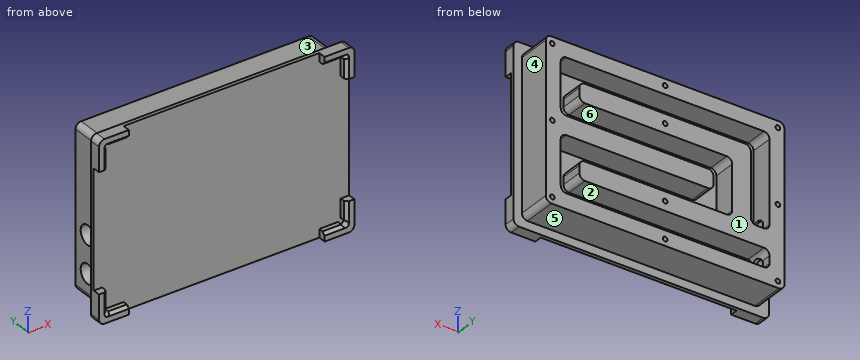
```python
from build123d import *

# Parameters (mm, degrees)
SKETCH1_W                         = 128
SKETCH1_H                         = 85.7
BOSS_EXTRUDE1_DEPTH               = 18
CUT_EXTRUDE1_DEPTH                = 12
M3X0_5_TAPPED_HOLE1_D             = 2.5
M3X0_5_TAPPED_HOLE1_DEPTH         = 10
M3X0_5_TAPPED_HOLE1_TIP           = 0.751075774
SKETCH10_W                        = 137
SKETCH10_H                        = 94.7
BOSS_EXTRUDE2_DEPTH               = 6
CUT_EXTRUDE2_DEPTH                = 4
SKETCH12_W                        = 4.5
SKETCH12_H                        = 62.7
SKETCH12_W_2                      = 105
SKETCH12_H_2                      = 4.475
CUT_EXTRUDE3_DEPTH                = 4
CHAMFER1_SIZE                     = 1.5
FILLET1_R                         = 3
F_1_8_NPT_TAPPED_HOLE1_AT_2_COUNT = 2
F_1_8_NPT_TAPPED_HOLE1_AT_2_PITCH = 19.935714286


with BuildPart() as part:
    # Sketch1 → Boss-Extrude1 (new body)
    with BuildSketch(Plane(origin=(0, 0, 0), x_dir=(1, 0, 0), z_dir=(0, 1, 0))):
        Rectangle(SKETCH1_W, SKETCH1_H)
    extrude(amount=BOSS_EXTRUDE1_DEPTH)

    # Sketch2 → Cut-Extrude1 (cut)
    with BuildSketch(Plane(origin=(0, 18, 0), x_dir=(1, 0, 0), z_dir=(0, 1, 0))):
        with BuildLine():
            Line((-46, 11.935714286), (-46, -21.892857143))
            ThreePointArc((-46, -21.892857143), (-45.121320344, -24.014177486), (-43, -24.892857143))
            Line((-43, -24.892857143), (43, -24.892857143))
            ThreePointArc((43, -24.892857143), (45.121320344, -24.014177486), (46, -21.892857143))
            Line((46, -21.892857143), (46, -17.935714286))
            ThreePointArc((46, -17.935714286), (45.121320344, -15.814393942), (43, -14.935714286))
            Line((43, -14.935714286), (-33, -14.935714286))
            ThreePointArc((-33, -14.935714286), (-35.121320344, -14.057034629), (-36, -11.935714286))
            Line((-36, -11.935714286), (-36, 11.935714286))
            ThreePointArc((-36, 11.935714286), (-35.121320344, 14.057034629), (-33, 14.935714286))
            Line((-33, 14.935714286), (43, 14.935714286))
            ThreePointArc((43, 14.935714286), (45.121320344, 15.814393942), (46, 17.935714286))
            Line((46, 17.935714286), (46, 21.892857143))
            ThreePointArc((46, 21.892857143), (45.121320344, 24.014177486), (43, 24.892857143))
            Line((43, 24.892857143), (-53, 24.892857143))
            ThreePointArc((-53, 24.892857143), (-55.121320344, 25.771536799), (-56, 27.892857143))
            Line((-56, 27.892857143), (-56, 31.85))
            ThreePointArc((-56, 31.85), (-55.121320344, 33.971320344), (-53, 34.85))
            Line((-53, 34.85), (53, 34.85))
            ThreePointArc((53, 34.85), (55.121320344, 33.971320344), (56, 31.85))
            Line((56, 31.85), (56, 7.978571429))
            ThreePointArc((56, 7.978571429), (55.121320344, 5.857251085), (53, 4.978571429))
            Line((53, 4.978571429), (-23, 4.978571429))
            ThreePointArc((-23, 4.978571429), (-25.121320344, 4.099891772), (-26, 1.978571429))
            Line((-26, 1.978571429), (-26, -1.978571429))
            ThreePointArc((-26, -1.978571429), (-25.121320344, -4.099891772), (-23, -4.978571429))
            Line((-23, -4.978571429), (53, -4.978571429))
            ThreePointArc((53, -4.978571429), (55.121320344, -5.857251085), (56, -7.978571429))
            Line((56, -7.978571429), (56, -31.85))
            ThreePointArc((56, -31.85), (55.121320344, -33.971320344), (53, -34.85))
            Line((53, -34.85), (-53, -34.85))
            ThreePointArc((-53, -34.85), (-55.121320344, -33.971320344), (-56, -31.85))
            Line((-56, -31.85), (-56, 11.935714286))
            ThreePointArc((-56, 11.935714286), (-55.121320344, 14.057034629), (-53, 14.935714286))
            Line((-53, 14.935714286), (-49, 14.935714286))
            ThreePointArc((-49, 14.935714286), (-46.878679656, 14.057034629), (-46, 11.935714286))
        make_face()
    extrude(amount=-CUT_EXTRUDE1_DEPTH, mode=Mode.SUBTRACT)

    # M3x0.5 Tapped Hole1
    with Locations(Plane(origin=(0, 18, 0), x_dir=(1, 0, 0), z_dir=(0, 1, 0))):
        with Locations((-60.5, 39.35), (0, 39.35), (60.5, 39.35), (60.5, 0), (60.5, -39.35), (0, -39.35), (-60.5, -39.35), (-60.5, 0), (0, 19.914285714), (0, -19.914285714)):
            Hole(M3X0_5_TAPPED_HOLE1_D / 2, depth=M3X0_5_TAPPED_HOLE1_DEPTH)
            with Locations((0, 0, -(M3X0_5_TAPPED_HOLE1_DEPTH + M3X0_5_TAPPED_HOLE1_TIP / 2))):  # 118° drill point
                Cone(0, M3X0_5_TAPPED_HOLE1_D / 2, M3X0_5_TAPPED_HOLE1_TIP, mode=Mode.SUBTRACT)

    # Sketch10 → Boss-Extrude2 (add)
    with BuildSketch(Plane.XZ):
        Rectangle(SKETCH10_W, SKETCH10_H)
    extrude(amount=BOSS_EXTRUDE2_DEPTH)

    # Sketch11 → Cut-Extrude2 (cut)
    with BuildSketch(Plane.XZ.offset(6)):
        with BuildLine():
            Line((-62.5, -42.875), (62.5, -42.875))
            ThreePointArc((62.5, -42.875), (65.060660172, -43.935660172), (64, -41.375))
            Line((64, -41.375), (64, 41.375))
            ThreePointArc((64, 41.375), (65.060660172, 43.935660172), (62.5, 42.875))
            Line((62.5, 42.875), (-62.5, 42.875))
            ThreePointArc((-62.5, 42.875), (-65.060660172, 43.935660172), (-64, 41.375))
            Line((-64, 41.375), (-64, -41.375))
            ThreePointArc((-64, -41.375), (-65.060660172, -43.935660172), (-62.5, -42.875))
        make_face()
    extrude(amount=-CUT_EXTRUDE2_DEPTH, mode=Mode.SUBTRACT)

    # Sketch12 → Cut-Extrude3 (cut)
    with BuildSketch(Plane.XZ.offset(6)):
        with Locations((-66.25, 0)):
            Rectangle(SKETCH12_W, SKETCH12_H)
        with Locations((66.25, 0)):
            Rectangle(SKETCH12_W, SKETCH12_H)
        with Locations((0, 45.1125)):
            Rectangle(SKETCH12_W_2, SKETCH12_H_2)
        with Locations((0, -45.1125)):
            Rectangle(SKETCH12_W_2, SKETCH12_H_2)
    extrude(amount=-CUT_EXTRUDE3_DEPTH, mode=Mode.SUBTRACT)

    # Chamfer1
    chamfer1_edges = [part.edges().sort_by_distance(p)[0] for p in [
        (-64, -6, 36.3625),
        (-57.5, -6, -42.875),
        (64, -6, -36.3625),
        (57.5, -6, 42.875),
        (-64, -6, -36.3625),
        (57.5, -6, -42.875),
        (64, -6, 36.3625),
        (-57.5, -6, 42.875),
    ]]
    chamfer(chamfer1_edges, length=CHAMFER1_SIZE - 0.0001)  # a hair under: the kernel refuses the full size

    # Fillet1
    fillet1_edges = [part.edges().sort_by_distance(p)[0] for p in [
        (-68.5, -3, -47.35),
        (68.5, -3, -47.35),
        (68.5, -3, 47.35),
        (-68.5, -3, 47.35),
        (64, 9, 42.85),
        (-64, 9, 42.85),
        (-64, 9, -42.85),
        (64, 9, -42.85),
    ]]
    fillet(fillet1_edges, radius=FILLET1_R)

    # Sketch14 → 1/8 NPT Tapped Hole1 (revolve, cut)
    with BuildSketch(Plane(origin=(-64, 9, -29.871428571), x_dir=(0, 0, 1), z_dir=(0, 1, 0))):
        Polygon((0, 0), (0, 14.153468714), (4.2164, 11.62), (4.2164, 6.92), (4.936178933, 6.92), (5.143373, 0), align=None)
    f_1_8_npt_tapped_hole1 = revolve(axis=Axis((-70.35, 9, -29.871428571), (1, 0, 0)), mode=Mode.SUBTRACT)

    # 1/8 NPT Tapped Hole1 at 2: 1/8 NPT Tapped Hole1 ×2
    with Locations(*[(0, 0, i * F_1_8_NPT_TAPPED_HOLE1_AT_2_PITCH) for i in range(1, F_1_8_NPT_TAPPED_HOLE1_AT_2_COUNT)]):
        add(f_1_8_npt_tapped_hole1, mode=Mode.SUBTRACT)


solid = part.part
```
Input: part model. Units: mm. Frame: model coordinates. Face numbers are marked on the shaded views. A direction names the side the tool comes from. Coordinates: 2 decimals unless noted, no trailing zeros. Write each loop counter-clockwise with the first axis right and the second up, starting at its lowest first coordinate (ties: lowest second). Pieces come first, ordered by that corner, then holes.
1) Section A-A on x = 22.5. Output: boundary loops of the cut face in (y, z).
2) Section C-C on x = -29. Output: boundary loops of the cut face in (y, z), and give its area (3 significant figures).
3) Section B-B on y = 15.5. State how many separate pieces and enclosed holes the cut face has, and give its area (3 significant figures).
4) Set-up query: the marked faces 1 and 2. Return all of +Z, -Z, +X, -X, +Y, -Y with unobstructed straight access to the full face (end or side cutting, diameter ignored); none if empty.
5) Pin query (flat end, axial travel): pin 1 Ø2 at (x, z) = (-60.5, 0) entering from +Y; pin 2 Ø3 at (x, z) = (0, -19.91) entering from -Y; pin 3 Ø9.5 at (x, y) = (13, 9) entering from +Z. Return the tip coordinate at first contact, or that it passes through.
6) Mould query, pull axis Z, two halves, no side actions, for the marked faces 3, 4, 5 and 6. Classes: pulls with the +Z half, pulls with the -Z half, needs draft (parallel to the pull), parting line crosses it, or undercut.
7) Material intervals for line 1 along Z through (x, y) = (-60.5, 15.25); line 2 along Z through (x, y) = (40.5, 9); line 3 along Z through (x, y) = (-52, 10.5), sorted ascending.
Check result:
1. outline: (-2, -47.35) - (0, -47.35) - (0, -42.85) - (18, -42.85) - (18, -34.85) - (6, -34.85) - (6, -24.89) - (18, -24.89) - (18, -14.94) - (6, -14.94) - (6, -4.98) - (18, -4.98) - (18, 4.98) - (6, 4.98) - (6, 14.94) - (18, 14.94) - (18, 24.89) - (6, 24.89) - (6, 34.85) - (18, 34.85) - (18, 42.85) - (0, 42.85) - (0, 47.35) - (-2, 47.35) - close
2. outline: (-2, -47.35) - (0, -47.35) - (0, -42.85) - (18, -42.85) - (18, -34.85) - (6, -34.85) - (6, -24.89) - (18, -24.89) - (18, -14.94) - (6, -14.94) - (6, 14.94) - (18, 14.94) - (18, 24.89) - (6, 24.89) - (6, 34.85) - (18, 34.85) - (18, 42.85) - (0, 42.85) - (0, 47.35) - (-2, 47.35) - close
2. area: 1,130 mm2
3. separate pieces: 1
3. enclosed holes: 11
3. area: 6,160 mm2
4. face 1: +Z, -Z, +X, -X, +Y
4. face 2: +Y
5. pin 1: stops at y = 7.85
5. pin 2: stops at y = -2
5. pin 3: stops at z = 42.85
6. face 3: pulls with the +Z half
6. face 4: needs draft
6. face 5: pulls with the -Z half
6. face 6: undercut
7. line 1: z = -42.85 to -40.6, -38.1 to -1.25, 1.25 to 38.1, 40.6 to 42.85
7. line 2: z = -42.85 to -34.85, -24.89 to -14.94, -4.98 to 4.98, 14.94 to 24.89, 34.85 to 42.85
7. line 3: z = -42.85 to -34.85, -24.89 to -14.94, 34.85 to 42.85
